Geometry: final body of the model. Coordinates: model frame, mm. Give positions to 0.01 mm unless a question says otherwise; leave off trailing zeros. Write each loop counter-clockwise with the first axis right and the second up, starting at its lowest first coordinate (ties: lowest second). Pieces come first, ordered by that corner, then holes. Notation, with made-up numbers: (18.5, 25) -> (28.5, 25) arc R26 cw to (28.5, 52) -> close; hole circle Ø7 at (79, -9). An arc over 180 degrees is marked (long way). Answer as a JSON object with one key per item and string values.
from build123d import *

# Parameters (mm, degrees)
F0_W     = 56
F0_H     = 87.6
F1_DEPTH = 3
F2_SIZE  = 2
F3_W     = 15.5
F3_H     = 25
F4_DEPTH = 1
F5_R     = 3
F8_D     = 2.5
F8_DEPTH = 68
F8_TIP   = 0.7510757738


with BuildPart() as f1:
    # F0 (on Top) → F1 (new body)
    with BuildSketch(Plane.XY):
        Rectangle(F0_W, F0_H)
    extrude(amount=F1_DEPTH)

    # F2
    f2_edges = [f1.edges().sort_by_distance(p)[0] for p in [
        (-28, 0, 0),
    ]]
    chamfer(f2_edges, length=F2_SIZE)

    # F3 (on face) → F4 (cut)
    with BuildSketch(Plane.XY.offset(3)):
        Polygon((12.5, 43.8), (-12.5, 43.8), (-12.5, -43.8), (12.5, -43.8), (12.5, -12.5), (12.5, 12.5), align=None)
        with Locations((20.25, 0)):
            Rectangle(F3_W, F3_H)
    extrude(amount=-F4_DEPTH, mode=Mode.SUBTRACT)

    # F5
    f5_edges = [f1.edges().sort_by_distance(p)[0] for p in [
        (-28, 43.8, 2.5),
        (-28, -43.8, 2.5),
        (28, -43.8, 1.5),
        (28, 43.8, 1.5),
    ]]
    fillet(f5_edges, radius=F5_R)

    # F8
    with Locations(Plane.XY.offset(3)):
        with Locations((-20, 35.8), (20, 35.8), (20, 17.5), (20, -17.5), (20, -35.8), (-20, -35.8), (-20, 17.5), (-20, -17.5)):
            Hole(F8_D / 2, depth=F8_DEPTH)
            with Locations((0, 0, -(F8_DEPTH + F8_TIP / 2))):  # 118° drill point
                Cone(0, F8_D / 2, F8_TIP, mode=Mode.SUBTRACT)


solid = f1.part
Q1. Cut plane D-D (y = 28). Return the cut outline in (x, z).
Values:
{"outline": "(-28, 2) -> (-26, 0) -> (28, 0) -> (28, 3) -> (12.5, 3) -> (12.5, 2) -> (-12.5, 2) -> (-12.5, 3) -> (-28, 3) -> close"}
Q2. First-contact query: P1, Ø2, axis at x = 20, y = -35.8, coming from the -Z side; P2, Ø3, axis at x = 6.5, y = -23, coming from the +Z side; P3, Ø0.5, axis at y = -11, z = 2.5, coming from the +X side. Flat tips, straight axial feed; report the tip coordinate or a pass-through.
Values:
{"P1": "through", "P2": "z = 2", "P3": "x = -12.5"}
Q3. Material intervals for L1, parallel to Y at x = 20, z = 0.1; L2, parallel to Y at x = 14, z = 2.25; L3, parallel to X at y = 16, z = 2.8, sorted ascending. Write a range as from..to.
Values:
{"L1": "-43.8..-37.05, -34.55..-18.75, -16.25..16.25, 18.75..34.55, 37.05..43.8", "L2": "-43.8..-12.5, 12.5..43.8", "L3": "-28..-12.5, 12.5..28"}
Q4. Mould query, pull axis X, two halves, no side actions, for faces 1 (the cylindrical face through (-26.748, -43.238, 1.854)), 2 (the cylindrical face through (20.16, 37.04, 1.48)), 3 (the flat face through (0, 43.8, 1)), 4 (the cylindrical face through (27.1, 42.94, 1.52)). Classes: pulls with the +X half, pulls with the -X half, needs draft (parallel to the pull), parting line crosses it, or undercut.
Values:
{"face 1": "pulls with the -X half", "face 2": "undercut", "face 3": "needs draft", "face 4": "pulls with the +X half"}
Q5. Cut plane A-A (z = 2.5). State how many separate pieces and enclosed holes the cut face has, and give its area (3 significant figures).
Values:
{"separate pieces": "3", "enclosed holes": "8", "area": "2,280 mm²"}
Q6. Cut plane C-C (y = -17.5). Return the cut outline in (x, z).
Values:
{"outline": "(-28, 2) -> (-26, 0) -> (-21.25, 0) -> (-21.25, 3) -> (-28, 3) -> close; (-18.75, 0) -> (18.75, 0) -> (18.75, 3) -> (12.5, 3) -> (12.5, 2) -> (-12.5, 2) -> (-12.5, 3) -> (-18.75, 3) -> close; (21.25, 0) -> (28, 0) -> (28, 3) -> (21.25, 3) -> close"}
Q7. Cut plane B-B (x = -20). Return the cut outline in (y, z), and give its area (3 significant figures).
Values:
{"outline": "(-43.8, 0) -> (-37.05, 0) -> (-37.05, 3) -> (-43.8, 3) -> close; (-34.55, 0) -> (-18.75, 0) -> (-18.75, 3) -> (-34.55, 3) -> close; (-16.25, 0) -> (16.25, 0) -> (16.25, 3) -> (-16.25, 3) -> close; (18.75, 0) -> (34.55, 0) -> (34.55, 3) -> (18.75, 3) -> close; (37.05, 0) -> (43.8, 0) -> (43.8, 3) -> (37.05, 3) -> close", "area": "233 mm²"}
